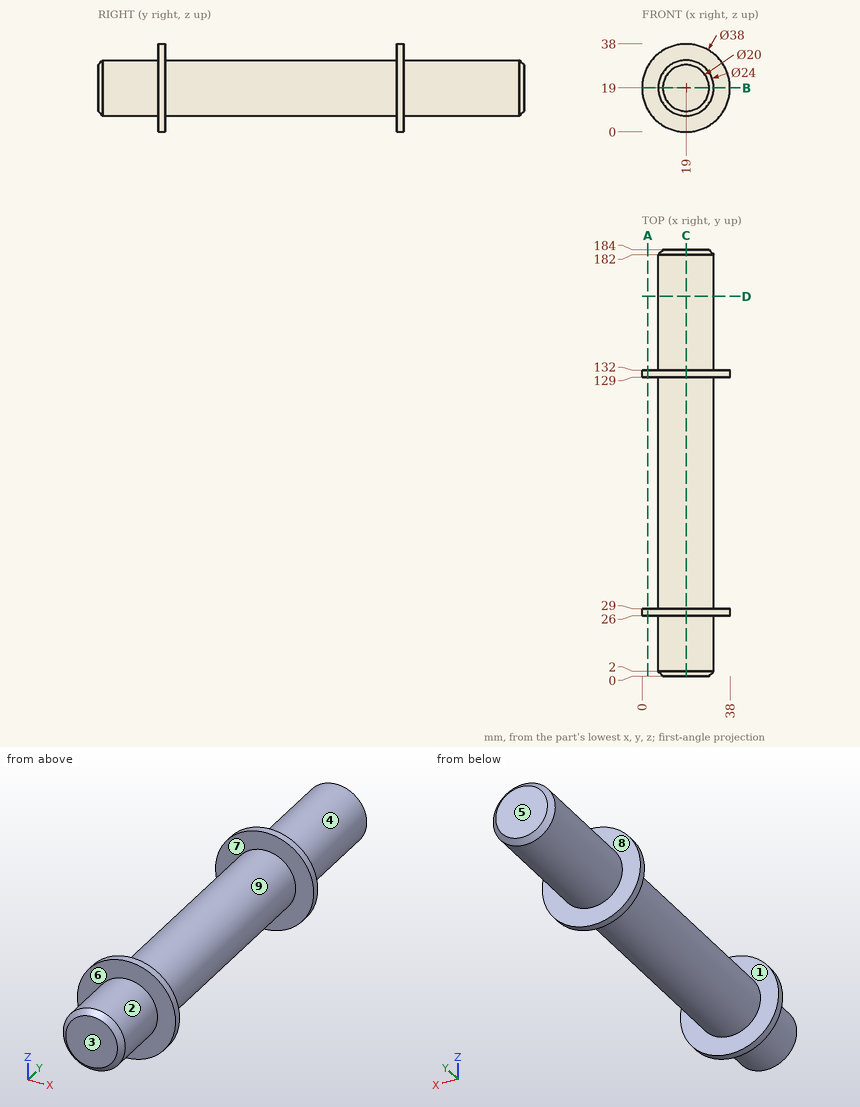
Can you work these out from the drawing? Everything is in mm from the part's minimum corner. A direction names the side the tool comes from. Coordinates: 2 decimals unless noted, no trailing zeros. Loops run counter-clockwise (first coordinate to the right, second up) from the corner with the lowest first, then second, coordinate; pieces in that order, holes last.
1) Please list where these lines run through material, in increasing order: line 1 along Y through (x, z) = (3.5, 20); line 2 along X through (y, z) = (28, 36.5); line 3 along X through (y, z) = (94, 14).
Reported:
line 1: y = 26 to 29, 129 to 132
line 2: x = 11.6 to 26.4
line 3: x = 8.09 to 29.91
2) Imagine slicing it at B-B (z = 19). List the corners of the cut face in (x, y) for me, and give its area (3 significant figures).
Reported:
outline: (0, 26) - (7, 26) - (7, 2) - (9, 0) - (29, 0) - (31, 2) - (31, 26) - (38, 26) - (38, 29) - (31, 29) - (31, 129) - (38, 129) - (38, 132) - (31, 132) - (31, 182) - (29, 184) - (9, 184) - (7, 182) - (7, 132) - (0, 132) - (0, 129) - (7, 129) - (7, 29) - (0, 29) - close
area: 4,490 mm2
3) Imagine slicing it at C-C (x = 19). List the corners of the cut face in (y, z) for me, and give its area (3 significant figures).
Reported:
outline: (0, 9) - (2, 7) - (26, 7) - (26, 0) - (29, 0) - (29, 7) - (129, 7) - (129, 0) - (132, 0) - (132, 7) - (182, 7) - (184, 9) - (184, 29) - (182, 31) - (132, 31) - (132, 38) - (129, 38) - (129, 31) - (29, 31) - (29, 38) - (26, 38) - (26, 31) - (2, 31) - (0, 29) - close
area: 4,490 mm2
4) Will these pins go through, and if not, where does the flat tip stop? pin 1 Ø8 at (y, z) = (94, 23) entering from +X; pin 2 Ø3 at (y, z) = (36, 27.5) entering from +X; pin 3 Ø2 at (x, y) = (30, 111.5) entering from +Z.
Reported:
pin 1: stops at x = 31
pin 2: stops at x = 28.75
pin 3: stops at z = 25.63
5) Which directions (+Z, -Z, +X, -X, +Y, -Y) give clear straight access to the entire face, cutting with the end or side of a thin tool? Please do the marked faces 1, 2, 3, 4 and 5.
Reported:
face 1: none
face 2: -Y
face 3: +Z, -Z, +X, -X, -Y
face 4: +Y
face 5: +Z, -Z, +X, -X, +Y
6) Thinking about a two-plate mould opening in Y: for the marked faces 6, 7, 8 and 9, which applies, released by +Y, released by -Y, zero draft, split by the parting line, or undercut?
Reported:
face 6: released by -Y
face 7: undercut
face 8: released by +Y
face 9: undercut
7) Imagine slicing it at A-A (x = 2.5). List the corners of the cut face in (y, z) for me.
Reported:
outline: (26, 9.58) - (29, 9.58) - (29, 28.42) - (26, 28.42) - close; (129, 9.58) - (132, 9.58) - (132, 28.42) - (129, 28.42) - close
8) Imagine slicing it at D-D (y = 164). List the corners of the cut face in (x, z) for me, and give its area (3 significant figures).
Reported:
outline: circle Ø24 at (19, 19)
area: 452 mm2
